```python
from build123d import *

# Parameters (mm, degrees)
SKETCH_1_R      = 11.1
SKETCH_1_R_2    = 1.8
SKETCH_1_R_3    = 4.5
SKETCH_1_R_4    = 1.5
EXTRUDE_1_DEPTH = 3
FILLET_1_R      = 1.5
FILLET_2_R      = 7
FILLET_3_R      = 4


with BuildPart() as part:
    # 草图1 → 凸台-拉伸1 (new body)
    with BuildSketch(Plane.XY):
        with BuildLine():
            Line((-5, 21.8), (-5, 29))
            ThreePointArc((-5, 29), (0, 34), (5, 29))
            Line((5, 29), (5, 21.8))
            Line((5, 21.8), (39, 21.8))
            Line((39, 21.8), (39, -21.8))
            Line((39, -21.8), (-39, -21.8))
            Line((-39, -21.8), (-39, 21.8))
            Line((-39, 21.8), (-5, 21.8))
        make_face()
        Circle(SKETCH_1_R, mode=Mode.SUBTRACT)
        with Locations((0, 29)):
            Circle(SKETCH_1_R_2, mode=Mode.SUBTRACT)
        with Locations((25.11473671, -14.5)):
            Circle(SKETCH_1_R_2, mode=Mode.SUBTRACT)
        with Locations((-25.11473671, -14.5)):
            Circle(SKETCH_1_R_2, mode=Mode.SUBTRACT)
        with Locations((0, 19.25)):
            Circle(SKETCH_1_R_3, mode=Mode.SUBTRACT)
        with Locations((35, 16.8)):
            Circle(SKETCH_1_R_4, mode=Mode.SUBTRACT)
        with Locations((35, -16.8)):
            Circle(SKETCH_1_R_4, mode=Mode.SUBTRACT)
        with Locations((-35, 16.8)):
            Circle(SKETCH_1_R_4, mode=Mode.SUBTRACT)
        with Locations((-35, -16.8)):
            Circle(SKETCH_1_R_4, mode=Mode.SUBTRACT)
        Polygon((11.856406461, 11.464101615), (15.856406461, 4.535898385), (20.186533479, 7.035898385), (16.186533479, 13.964101615), align=None, mode=Mode.SUBTRACT)
    extrude(amount=EXTRUDE_1_DEPTH)

    # 圆角1
    fillet_1_edges = [part.edges().sort_by_distance(p)[0] for p in [
        (16.186533479, 13.964101615, 1.5),
        (11.856406461, 11.464101615, 1.5),
        (15.856406461, 4.535898385, 1.5),
        (20.186533479, 7.035898385, 1.5),
    ]]
    fillet(fillet_1_edges, radius=FILLET_1_R)

    # 圆角2
    fillet_2_edges = [part.edges().sort_by_distance(p)[0] for p in [
        (-5, 21.8, 1.5),
        (5, 21.8, 1.5),
    ]]
    fillet(fillet_2_edges, radius=FILLET_2_R)

    # 圆角3
    fillet_3_edges = [part.edges().sort_by_distance(p)[0] for p in [
        (39, 21.8, 1.5),
        (39, -21.8, 1.5),
        (-39, -21.8, 1.5),
        (-39, 21.8, 1.5),
    ]]
    fillet(fillet_3_edges, radius=FILLET_3_R)


solid = part.part
```
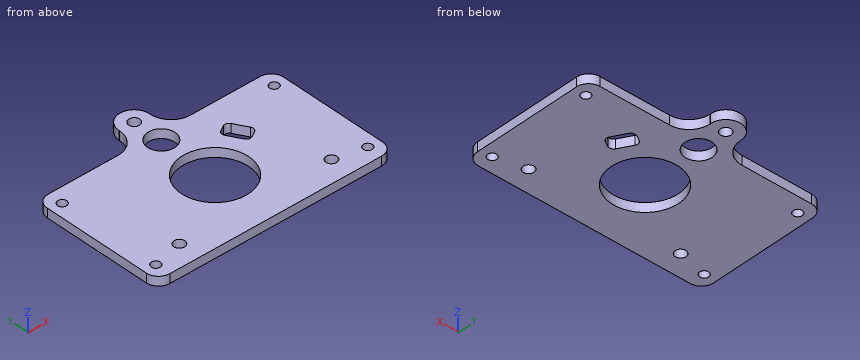
Geometry check sheet. Reference: the model listing, model coordinates, mm. Give positions to 0.01 mm unless a question says otherwise; leave off trailing zeros. Order: outer loops, then holes, each group sorted by start corner. A loop starts at its lowest first (then second) coordinate and runs counter-clockwise, first axis right, second up. Notation, with made-up numbers: (-23, 82.5) - (-15, 82.5) arc R27 cw to (-15, 98.5) - close; hole circle Ø6 at (39.25, 66). An arc over 180 degrees is marked (long way). Write item = value, one per line. Start each with the question number.
1) Section check C-C (z = 1.1). Count the separate pieces of the cut face and the enclosed holes in it, then the cut area to 3 significant figures.
2) Section check B-B (y = -14.5). Enter the section's corners in (x, z).
3) Section check D-D (y = 19.25). Enter the section's corners in (x, z), then the cut area to 3 significant figures.
4) Scan lines: L1, parallel to Y at x = 0, z = 1.7; L2, parallel to Y at x = 35, z = 1.4; L3, parallel to X at y = 10, z = 1.95. Record each from-to range of solid material in increasing order.
5) Section check A-A (x = 0). Enter the section's corners in (y, z), then the cut area to 3 significant figures.
6) Gauge pin test, flat ends, axial feed: pin 1 Ø4 at (x, y) = (35, 16.8) entering from +Z; pin 2 Ø1.5 at (x, z) = (7, 2) entering from +Y; pin 3 Ø3 at (x, y) = (0, 29) entering from -Z. Record the tip position at first contact, or that the pin passes through.
Geometry check:
q1.separate_pieces = 1
q1.enclosed_holes = 10
q1.area = 2,970 mm2
q2.outline = (-39, 0) - (-26.91, 0) - (-26.91, 3) - (-39, 3) - close; (-23.31, 0) - (23.31, 0) - (23.31, 3) - (-23.31, 3) - close; (26.91, 0) - (39, 0) - (39, 3) - (26.91, 3) - close
q3.outline = (-38.73, 0) - (-4.5, 0) - (-4.5, 3) - (-38.73, 3) - close; (4.5, 0) - (38.73, 0) - (38.73, 3) - (4.5, 3) - close
q3.area = 205 mm2
q4.L1 = -21.8 to -11.1, 11.1 to 14.75, 23.75 to 27.2, 30.8 to 34
q4.L2 = -21.8 to -18.3, -15.3 to 15.3, 18.3 to 21.8
q4.L3 = -39 to -4.82, 4.82 to 12.7, 18.48 to 39
q5.outline = (-21.8, 0) - (-11.1, 0) - (-11.1, 3) - (-21.8, 3) - close; (11.1, 0) - (14.75, 0) - (14.75, 3) - (11.1, 3) - close; (23.75, 0) - (27.2, 0) - (27.2, 3) - (23.75, 3) - close; (30.8, 0) - (34, 0) - (34, 3) - (30.8, 3) - close
q5.area = 63.0 mm2
q6.pin_1 = 3
q6.pin_2 = 24.81
q6.pin_3 = through
